Check sheet for the drawn part. Datum: minimum x, y, z corner. Units: mm. Round coordinates to 2 decimals unless told otherwise and drop trailing zeros. Write each loop counter-clockwise with the first axis right and the second up, starting at its lowest first coordinate (ties: lowest second). Pieces come first, ordered by that corner, then holes. Notation, with made-up numbers: M -25.5,56.5 L -6.5,56.5 A16 cw -6.5,80.5 Z; hole C 44,-25.75 d3. An arc over 180 degrees is marked long. Use a Markdown table: item, result.
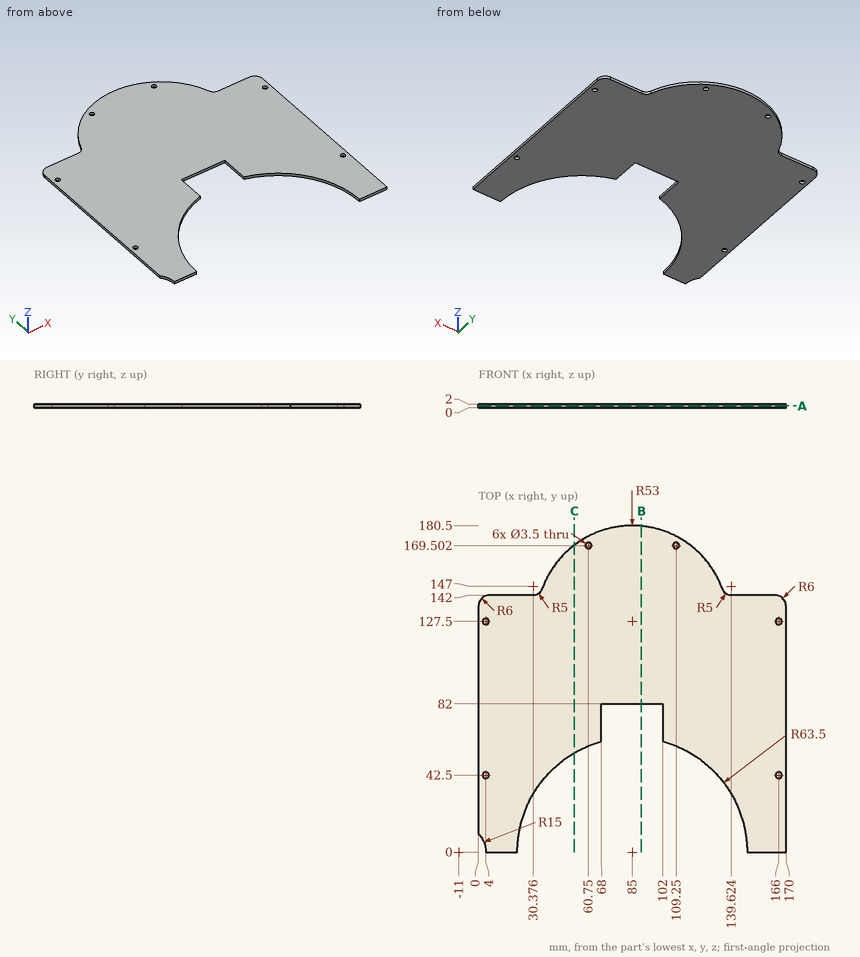
Item 1: Cross-section at A-A, the plane z = 1. Count the separate pieces of the cut face and the enclosed holes in it, and give its area (4 significant figures).
Outcome:
| item | result |
|---|---|
| separate pieces | 1 |
| enclosed holes | 6 |
| area | 19,950 mm2 |
Item 2: Cross-section at B-B, the plane x = 90. Record the cut outline in (y, z).
Outcome:
| item | result |
|---|---|
| outline | M 82,0 L 180.26,0 L 180.26,2 L 82,2 Z |
Item 3: Cross-section at C-C, the plane x = 53. Record the cut outline in (y, z), and give its area (3 significant figures).
Outcome:
| item | result |
|---|---|
| outline | M 54.85,0 L 169.75,0 L 169.75,2 L 54.85,2 Z |
| area | 230 mm2 |
Item 4: Material ranges on line 1 along X through (y, z) = (127.5, 1.2); line 2 along X through (y, z) = (170, 1) (1 decimal); line 3 along Y through (x, z) = (166, 1.1), recorded low to high. Write a range as from..to.
Outcome:
| item | result |
|---|---|
| line 1 | x = 0..2.25, 5.75..164.25, 167.75..170 |
| line 2 | x = 53.3..59.1, 62.4..107.6, 110.9..116.7 |
| line 3 | y = 0..40.75, 44.25..125.75, 129.25..141.66 |
Item 5: Go/stop test with flat-tipped pins: pin 1 (3 mm diameter, centred on x = 4, y = 42.5, fed in from +Z); pin 2 (1 mm diameter, centred on x = 137, z = 1.5, fed in from -Y). Record where each tip stops, or that it passes through.
Outcome:
| item | result |
|---|---|
| pin 1 | passes through |
| pin 2 | stops at y = 35.72 |
